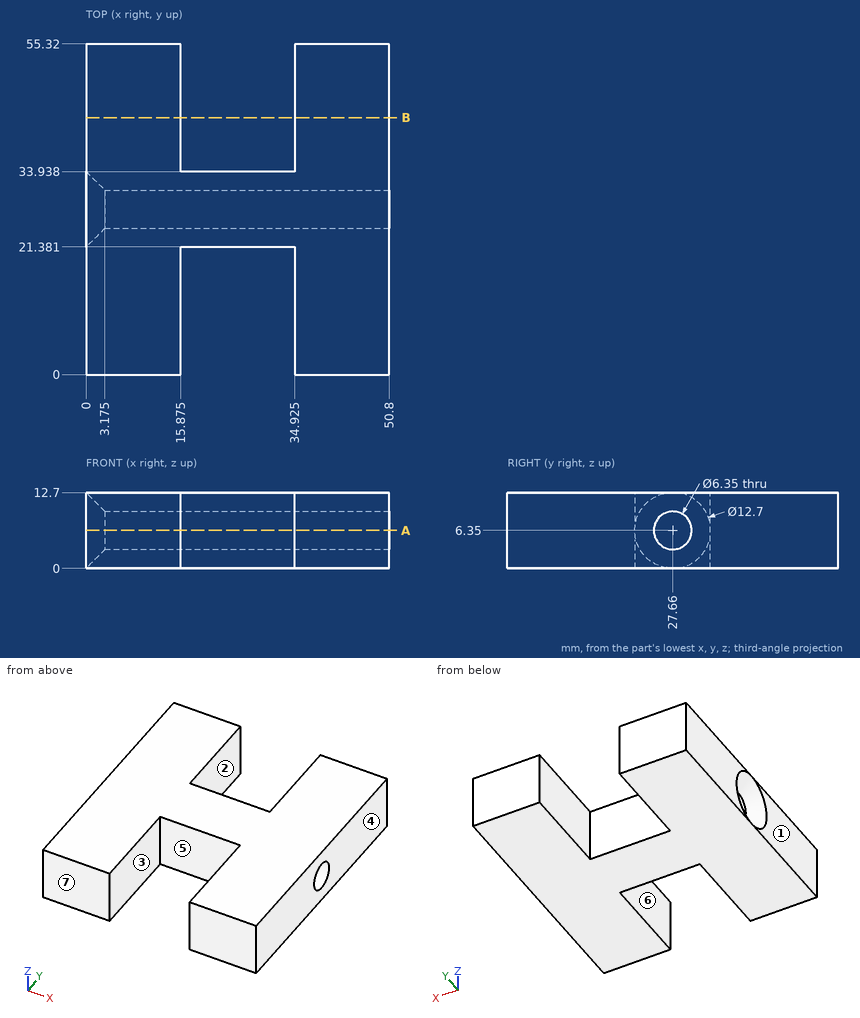
Source: three-view drawing plus pictorial views. Frame: mm from the lowest corner of the part. A direction names the side the tool comes from. Round coordinates to 2 decimals unless told otherwise and drop trailing zeros. Loops run counter-clockwise (first coordinate to the right, second up) from the corner with the lowest first, then second, coordinate; pieces in that order, holes last. Notation, with made-up numbers: M 19,67 L 47,67 A22 cw 47,100 Z; hole C 28,70 d1. An arc over 180 degrees is marked long. Put each result on its own line as item: value. Start each with the question number.
(1) Set-up query: the marked faces 1, 2 and 3. Return all of +Z, -Z, +X, -X, +Y, -Y with unobstructed straight access to the full face (end or side cutting, diameter ignored); none if empty.
(2) Material intervals for line 1 along Y through (x, z) = (40, 6.35) (1 decimal); line 2 along X through (y, z) = (15, 2.75) (1 decimal); line 3 along Y through (x, z) = (32, 6.35) (1 decimal), sorted ascending. Write a range as [from, to].
(3) Section query A-A (z = 6.35). Return loops of the section in (x, y) (1 decimal), then the cut area to 3 significant figures.
(4) Contact query for a flat-ended pin moving along its axis: pin 1 Ø6.5 at (x, z) = (29.5, 6) entering from -Y. Output: stop coordinate, or through.
(5) Section query B-B (y = 43). Return loops of the section in (x, z) (1 decimal).
(6) Draft query along X for the marked faces 4, 5, 6 and 7. Return one class per face: +X half, -X half, draft (parallel to the pull), parting line (faces both ways), or undercut.
Findings below:
1. face 1: +Z, -Z, -X, +Y, -Y
1. face 2: +Z, -Z, +Y
1. face 3: +Z, -Z, -Y
2. line 1: y = [0, 24.5], [30.8, 55.3]
2. line 2: x = [0, 15.9], [34.9, 50.8]
2. line 3: y = [21.4, 24.5], [30.8, 33.9]
3. outline: M 0,0 L 15.9,0 L 15.9,21.4 L 34.9,21.4 L 34.9,0 L 50.8,0 L 50.8,24.5 L 3.2,24.5 L 0,21.3 Z; M 0,34 L 3.2,30.8 L 50.8,30.8 L 50.8,55.3 L 34.9,55.3 L 34.9,33.9 L 15.9,33.9 L 15.9,55.3 L 0,55.3 Z
3. area: 1,660 mm2
4. pin 1: stops at y = 21.38
5. outline: M 0,0 L 15.9,0 L 15.9,12.7 L 0,12.7 Z; M 34.9,0 L 50.8,0 L 50.8,12.7 L 34.9,12.7 Z
6. face 4: +X half
6. face 5: undercut
6. face 6: undercut
6. face 7: draft
